from build123d import *

# Parameters (mm, degrees)
EXTRUDE_1_DEPTH         = 3
SKETCH_2_R              = 1.35
CUT_EXTRUDE_1_DEPTH     = 2.444444444
SKETCH_3_R              = 1.35
CUT_EXTRUDE_2_DEPTH     = 0.555555556
HOLE_WIZARD_2_7_2_7_1_D = 2.7
SKETCH_6_R              = 1.6
CUT_EXTRUDE_3_DEPTH     = 64.035907885


with BuildPart() as part:
    # 草图1 → 凸台-拉伸1 (new body)
    with BuildSketch(Plane.XY.offset(3)):
        with BuildLine():
            Line((23.778016459, 8.467622986), (-52.596358319, 8.467622986))
            ThreePointArc((-52.596358319, 8.467622986), (-62.214907854, 3.590303351), (-52.451603626, -0.990377005))
            Line((-52.451603626, -0.990377005), (23.856567017, 0.468594516))
            ThreePointArc((23.856567017, 0.468594516), (27.777721585, 4.50700022), (23.778016459, 8.467622986))
        make_face()
    extrude(amount=-EXTRUDE_1_DEPTH)

    # 草图2 → 切除-拉伸1 (cut)
    with BuildSketch(Plane.XY.offset(3)):
        with Locations(Location((23.77801746, 4.467622995, 0), (0, 0, 180))):
            Circle(SKETCH_2_R)
    extrude(amount=-CUT_EXTRUDE_1_DEPTH, mode=Mode.SUBTRACT)

    # 草图3 → 切除-拉伸2 (cut)
    with BuildSketch(Plane(origin=(0, 0, 0), x_dir=(-1, 0, 0), z_dir=(0, 0, -1))):
        with Locations(Location((-23.778017455, 4.467823177, 0), (0, 0, 359.991504025))):
            Circle(SKETCH_3_R)
    extrude(amount=-CUT_EXTRUDE_2_DEPTH, mode=Mode.SUBTRACT)

    # Ø2.7 (2.7) 直径孔1 (through all)
    with Locations(Plane.XY.offset(3)):
        with Locations((-56.215609969, 3.682122995)):
            Hole(HOLE_WIZARD_2_7_2_7_1_D / 2)

    # 草图6 → 切除-拉伸3 (cut, through all)
    with BuildSketch(Plane.XY.offset(3)):
        with Locations((-56.215609969, 3.682122995)):
            Circle(SKETCH_6_R)
        with Locations((23.778017455, 4.467823177)):
            Circle(SKETCH_6_R)
    extrude(amount=-CUT_EXTRUDE_3_DEPTH, mode=Mode.SUBTRACT)


solid = part.part
Geometry: final body of the model. Coordinates: model frame, mm. A direction names the side the tool comes from. Coordinates: 2 decimals unless noted, no trailing zeros. Write each loop counter-clockwise with the first axis right and the second up, starting at its lowest first coordinate (ties: lowest second). Pieces come first, ordered by that corner, then holes. Notation, with made-up numbers: (58.5, 23.5) - (68.5, 23.5) arc R17 cw to (68.5, 54.5) - close; hole circle Ø3 at (19, -5.75). An arc over 180 degrees is marked (long way). Return JSON: item names as keys, results as strings.
Item 1: Line query: L1, parallel to X at y = 3, z = 1.1; L2, parallel to X at y = 5.5, z = 1.85; L3, parallel to X at y = 2.25, z = 1.55. Output: solid intervals per line, ascending.
Completed:
{"L1": "x = -62.18 to -57.66, -54.77 to 23.14, 24.41 to 27.5", "L2": "x = -61.93 to 22.56, 25 to 27.64", "L3": "x = -62.04 to -56.93, -55.5 to 27.11"}
Item 2: Section query C-C (x = 20.5). Output: boundary loops of the cut face in (y, z).
Completed:
{"outline": "(0.4, 0) - (8.47, 0) - (8.47, 3) - (0.4, 3) - close"}
Item 3: Section query B-B (z = 1.85). Output: boundary loops of the cut face in (x, y).
Completed:
{"outline": "(-52.6, 8.47) arc R6 ccw (long way) to (-52.45, -0.99) - (23.86, 0.47) arc R4 ccw to (23.78, 8.47) - close; hole circle Ø3.2 at (-56.22, 3.68); hole circle Ø3.2 at (23.78, 4.47)"}
Item 4: Section query A-A (x = -56.5). Output: boundary loops of the cut face in (y, z), and give its area (3 significant figures).
Completed:
{"outline": "(-2.31, 0) - (2.11, 0) - (2.11, 3) - (-2.31, 3) - close; (5.26, 0) - (9.68, 0) - (9.68, 3) - (5.26, 3) - close", "area": "26.5 mm2"}
Item 5: Pin query (flat end, axial travel): pin 1 Ø2.5 at (x, y) = (23.78, 4.47) entering from +Z; pin 2 Ø1.5 at (x, z) = (-10.5, 2) entering from +Y. Return the tip coordinate at first contact, or that it passes through.
Completed:
{"pin 1": "passes through", "pin 2": "stops at y = 8.47"}
Item 6: Reachability of faces 1 (the face through (-14, 8.468, 2)), 2 (the face through (22.51, 3.49, 1.52)) from +Z, -Z, +X, -X, +Y, -Y: full face, straight path, thin tool, end or side. Return the list, or none.
Completed:
{"face 1": "+Z, -Z, +X, +Y", "face 2": "+Z, -Z"}
Item 7: Section query D-D (x = -13). Output: boundary loops of the cut face in (y, z).
Completed:
{"outline": "(-0.24, 0) - (8.47, 0) - (8.47, 3) - (-0.24, 3) - close"}
